Answer from the drawing. Dimensions are ordinates in mm from the lowest x, y and z of the part. A direction names the side the tool comes from. Round coordinates to 2 decimals unless told otherwise and drop trailing zeros. Write each loop counter-clockwise with the first axis right and the second up, starting at its lowest first coordinate (ties: lowest second). Pieces come first, ordered by that corner, then holes. Notation, with made-up numbers: (36.5, 7) -> (51.5, 7) arc R18 ccw to (51.5, 12) -> close; hole circle Ø3 at (-7.5, 33.5). An arc over 180 degrees is marked (long way). Answer as a JSON object with one key per item and string values. Group by question number.
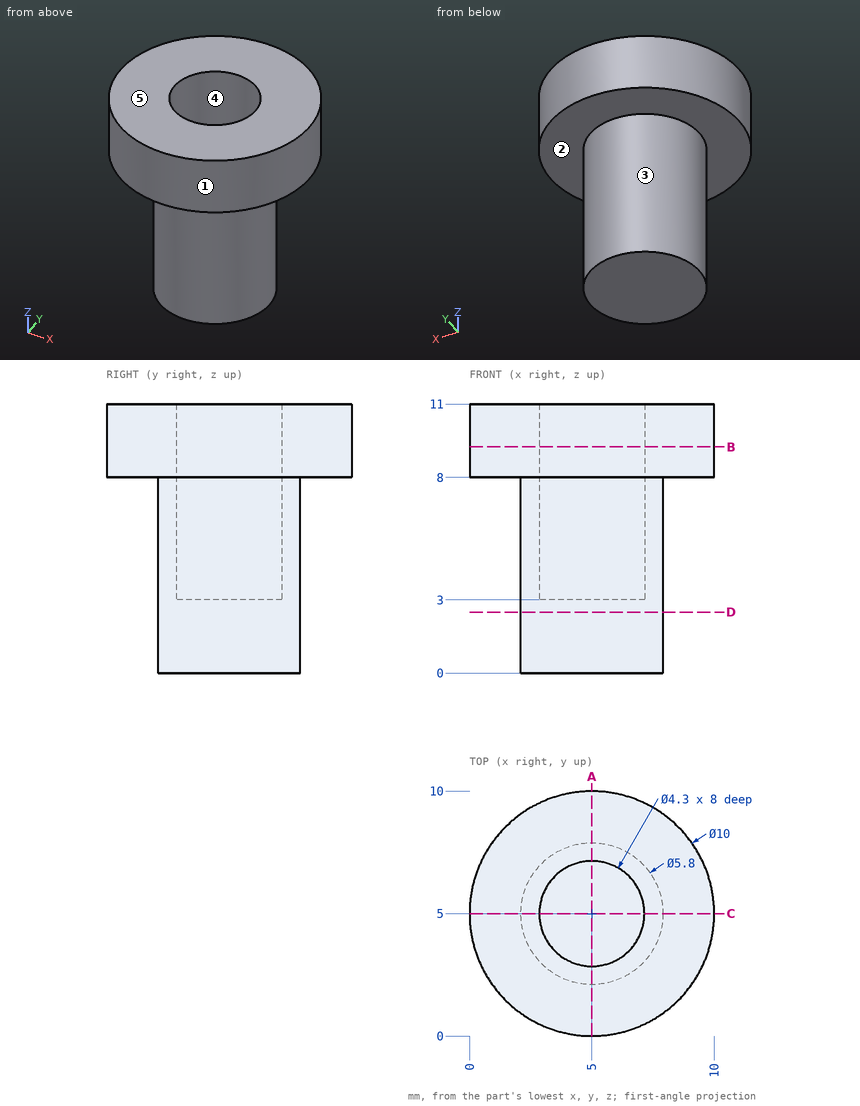
1) A cutting plane is placed at D-D on z = 2.5. Determine the outline of the cut face in (x, y), plus the area to 3 significant figures.
2) For a pull along X with two mould halves and no side action, classify the marked faces 3, 4 and 5 as released by +X, released by -X, zero draft, split by the parting line, or undercut.
3) Straight lines are drawn through the part: L1, parallel to Y at x = 5, z = 7.25; L2, parallel to Y at x = 5, z = 9.5; L3, parallel to Z at x = 3, y = 1.75. For each, find the intervals that lie inside material, in ascending order.
4) A tool of negligible diameter and unlimited length cuts with its end or side. For the marked faces 1 and 2, from which of +Z, -Z, +X, -X, +Y, -Y can it reach the whole face along a straight path? Write none if from no direction.
5) Each of these flat-tipped pins is pushed along its axis until it touches: P1, Ø4, axis at x = 5, y = 5, coming from the +Z side; P2, Ø3, axis at x = 1, z = 7.5, coming from the +Y side; P3, Ø1.5, axis at y = 1.5, z = 9.5, coming from the +X side. Where does it stop, or does it pass through?
6) A cutting plane is placed at A-A on x = 5. Determine the outline of the cut face in (y, z), plus the area to 3 significant figures.
7) A cutting plane is placed at B-B on z = 9.25. Determine the outline of the cut face in (x, y).
Established:
{
 "1": {"outline": "circle Ø5.8 at (5, 5)", "area": "26.4 mm²"},
 "2": {"face 3": "split by the parting line", "face 4": "undercut", "face 5": "zero draft"},
 "3": {"L1": "y = 2.1 to 2.85, 7.15 to 7.9", "L2": "y = 0 to 2.85, 7.15 to 10", "L3": "z = 8 to 11"},
 "4": {"face 1": "+Z, -Z", "face 2": "-Z"},
 "5": {"P1": "stops at z = 3", "P2": "stops at y = 9.28", "P3": "stops at x = 9.18"},
 "6": {"outline": "(0, 8) -> (2.1, 8) -> (2.1, 0) -> (7.9, 0) -> (7.9, 8) -> (10, 8) -> (10, 11) -> (7.15, 11) -> (7.15, 3) -> (2.85, 3) -> (2.85, 11) -> (0, 11) -> close", "area": "42.0 mm²"},
 "7": {"outline": "circle Ø10 at (5, 5); hole circle Ø4.3 at (5, 5)"}
}
